For this review, take the finished solid that the model builds, in its own axes (mm). Give positions to 0.01 mm unless a question says otherwise; leave off trailing zeros. Return JSON: item names as keys, results as strings. Group by question number.
1) Insertion check: P1, Ø7.5, axis at x = 101.6, z = 57.48, coming from the -Y side. The pin has a flat end and moves straight along its axis. Give the tip position at first contact, or say it passes through.
2) To check wall thickness, follow line 1 along Z through (x, y) = (0, -2); line 2 along Z through (x, y) = (-101.6, -4.4); line 3 along X through (y, z) = (-3.35, -5). State the ranges of each line that lie inside material, in increasing order.
3) The part is to be moulded in two halves that separate along Z. For faces 1 (the face through (-2, -3, 76.2)), 2 (the face through (2, 0, 1)), 3 (the face through (2, -3, -76.2)), 4 (the face through (104.76, -2.96, 56.78)), say which applies: released by +Z, released by -Z, zero draft, split by the parting line, or undercut.
Autodesk Inventor part; units mm, degrees
ref_plane "YZ Plane" through (0, 0, 0) normal (1, 0, 0) x (0, 1, 0)
ref_plane "XZ Plane" through (0, 0, 0) normal (0, 1, 0) x (-1, 0, 0)
ref_plane "XY Plane" through (0, 0, 0) normal (0, 0, 1) x (1, 0, 0)
sketch "Sketch1" plane through (0, 0, 0) normal (0, 1, 0) x (-1, 0, 0)
  line L0 (0, -106.68) -> (0, 106.68)
  line L1 (-177.8, 0) -> (177.8, 0)
  line L2 (-127, -76.2) -> (127, -76.2)
  line L3 (127, -76.2) -> (127, 76.2)
  line L4 (127, 76.2) -> (-127, 76.2)
  line L5 (-127, 76.2) -> (-127, -76.2)
  line L6 (-127, -76.2) -> (127, 76.2) construction
  line L7 (127, -76.2) -> (-127, 76.2) construction
  line L8 (101.6, 57.4802) -> (-101.6, 57.4802) construction
  line L9 (114.3, -6.35) -> (-114.3, -6.35) construction
  point P0 (0, 0)
  point P1 (0, -6.35)
  point P2 (63.5, -6.35)
  point P3 (-63.5, -6.35)
  dimension "d0" = 254
  dimension "d1" = 152.4
  dimension "d2" = 18.7198
  dimension "d3" = 101.6
  dimension "d4" = 101.6
  dimension "d5" = 82.55
  dimension "d6" = 114.3
  dimension "d7" = 12.7
  dimension "d28" = 50.8
  dimension "d29" = 50.8
extrude "Extrusion1" add sketch "Sketch1" against normal blind 5.842
hole "Hole1" at (-101.6, 0, 57.4802) at (101.6, 0, 57.4802) direction (0, -1, 0) diameter 6.477 end through all
hole "Hole2" at (-114.3, 0, -6.35) at (114.3, 0, -6.35) at (0, 0, -6.35) at (63.5, 0, -6.35) at (-63.5, 0, -6.35) direction (0, -1, 0) diameter 3.1242 end through all
pattern_linear "Rectangular Pattern1" count 2 spacing 53.975 along (0, 0, -1) of "Hole2"
sketch "Sketch2" plane through (0, 0, 0) normal (0, 1, 0) x (1, 0, 0)
  circle A0 centre (-114.3, 60.325) radius 1.5621
  circle A1 centre (-63.5, 60.325) radius 1.5621
  line L0 (-114.3, 60.325) -> (-63.5, 60.325) construction
  line L1 (-88.9, 60.325) -> (-88.9, 44.45) construction
  line L2 (-104.775, 45.0718) -> (-73.025, 45.0718) construction
  point P0 (0, 0)
  dimension "d31" = 31.75
  dimension "d32" = 15.875
  dimension "d33" = 15.875
hole "Hole3" at (-104.775, 0, -45.0718) at (-73.025, 0, -45.0718) direction (0, -1, 0) diameter 3.1242 end through all
fillet "Fillet1" radius 6.35 4 edges at (127, -2.921, 76.2) (127, -2.921, -76.2) (-127, -2.921, 76.2) (-127, -2.921, -76.2)
pattern_linear "Rectangular Pattern2" count 3 spacing 88.9 along (1, 0, 0) of "Hole3"
equation "\"d32\" = 0.5 * d31"
Evaluation:
{
 "1": {"P1": "y = -5.84"},
 "2": {"line 1": "-76.2 to -61.89, -58.76 to -7.91, -4.79 to 76.2", "line 2": "-76.2 to 54.24, 60.72 to 76.2", "line 3": "-127 to -115.09, -113.51 to -64.29, -62.71 to -0.79, 0.79 to 62.71, 64.29 to 113.51, 115.09 to 127"},
 "3": {"face 1": "released by +Z", "face 2": "zero draft", "face 3": "released by -Z", "face 4": "undercut"}
}
